The drawing under review shows one solid part. Ordinate dimensions are in mm from its lowest x, y, z. Round coordinates to 2 decimals unless told otherwise and drop trailing zeros. Loops run counter-clockwise (first coordinate to the right, second up) from the corner with the lowest first, then second, coordinate; pieces in that order, holes last. Notation, with made-up numbers: (29, -26) -> (57, -26) arc R18 cw to (57, 6) -> close; hole circle Ø2 at (39.5, 11.25). An arc over 180 degrees is marked (long way). Use a Markdown table: item, result. Add a question column.
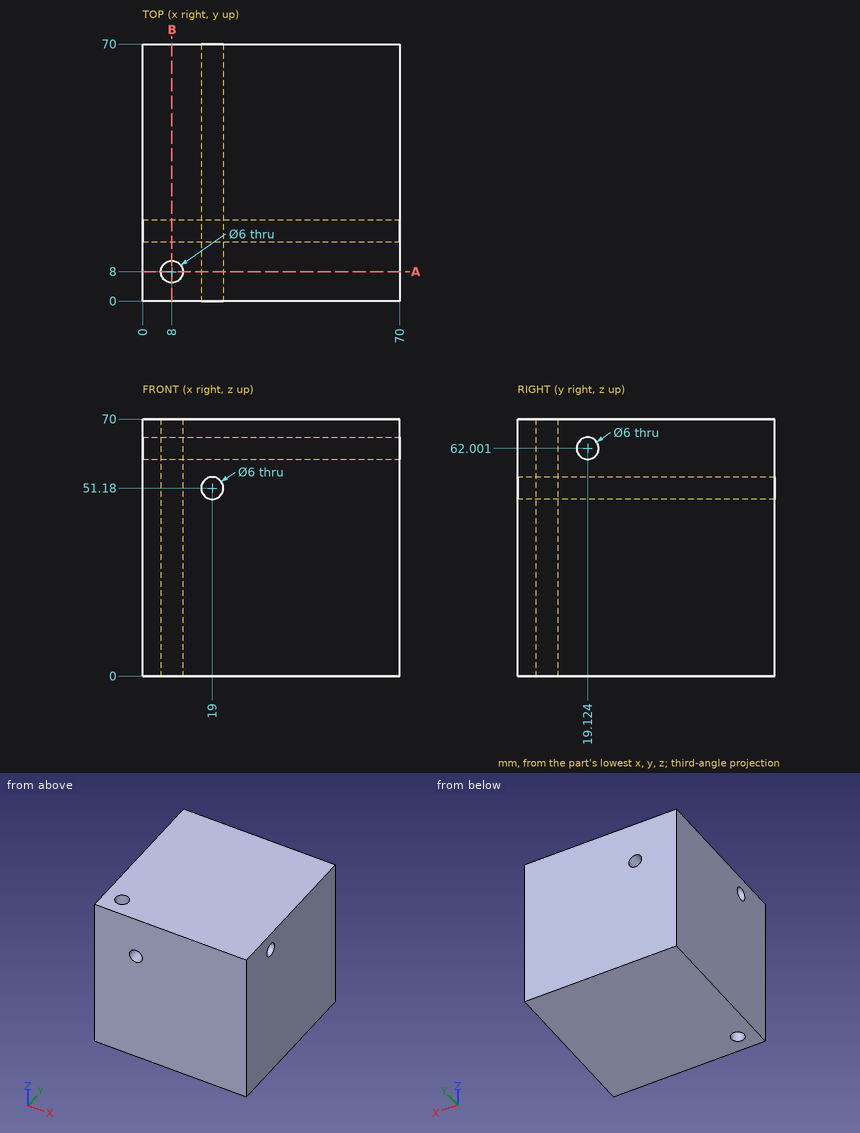
1. Consider section B-B on x = 8. State the section outline as (y, z) points (1 decimal).
2. To check wall thickness, follow probe 1 along X at (y, z) = (21.5, 51.5); probe 2 along Y at (x, z) = (8, 14). State the ranges of each line that lie inside material, in increasing order. Write a range as from..to.
3. Consider section A-A on y = 8. State the section outline as (x, z) points.
4. Insertion check: P1, Ø2, axis at x = 21, y = 30, coming from the -Z side; P2, Ø3.5, axis at x = 8, y = 8, coming from the +Z side. Each pin has a flat end and moves straight along its axis. Give the tip position at first contact, or say it passes through.
Verdict:
| question | item | result |
|---|---|---|
| 1 | outline | (0, 0) -> (5, 0) -> (5, 70) -> (0, 70) -> close; (11, 0) -> (70, 0) -> (70, 70) -> (11, 70) -> close; hole circle Ø6 at (19.1, 62) |
| 2 | probe 1 | x = 0..16.02, 21.98..70 |
| 2 | probe 2 | y = 0..5, 11..70 |
| 3 | outline | (0, 0) -> (5, 0) -> (5, 70) -> (0, 70) -> close; (11, 0) -> (70, 0) -> (70, 70) -> (11, 70) -> close; hole circle Ø6 at (19, 51.18) |
| 4 | P1 | stops at z = 0 |
| 4 | P2 | passes through |
